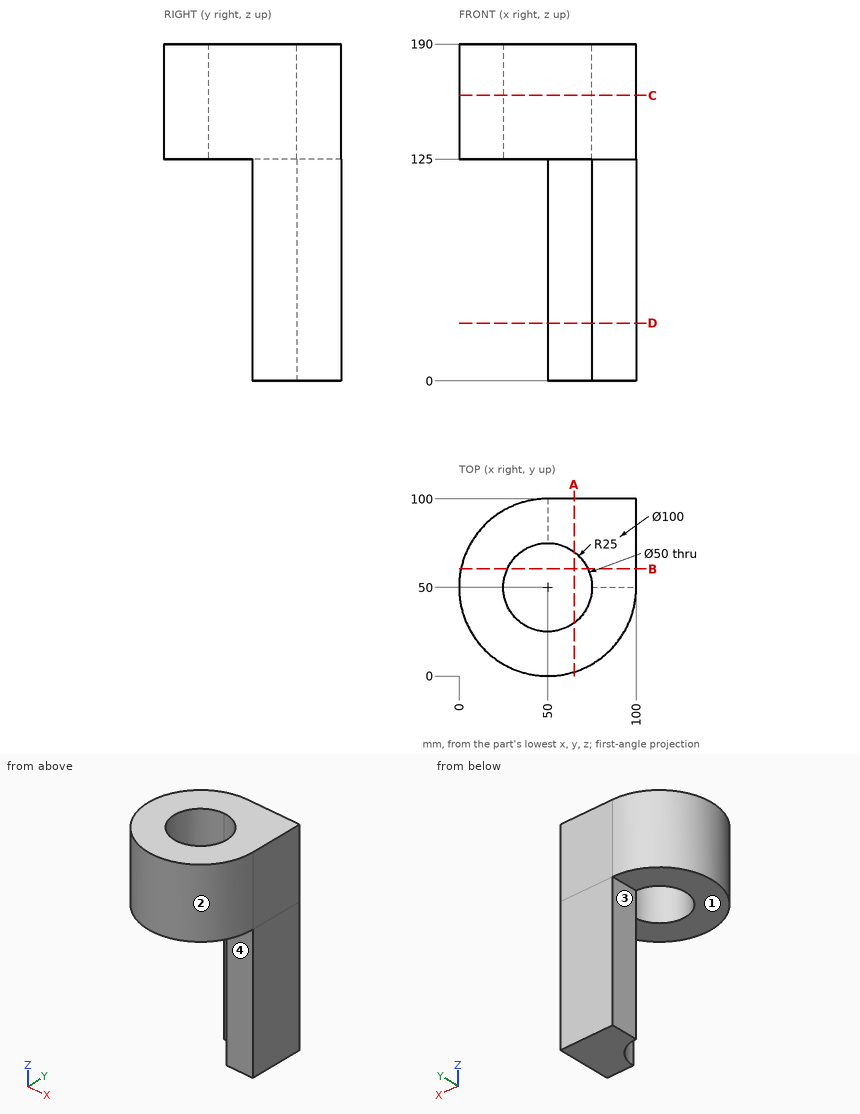
Could you check a few things on this drawing? It's one solid part, dimensions in mm from its lowest x, y, z. A direction names the side the tool comes from. Give positions to 0.01 mm unless a question says otherwise; leave off trailing zeros. Loops run counter-clockwise (first coordinate to the right, second up) from the corner with the lowest first, then second, coordinate; pieces in that order, holes last. Notation, with made-up numbers: M -29,-21 L -25,-21 A17 cw -25,-8 Z; hole C -36.75,85.5 d8. An arc over 180 degrees is marked long. Return JSON: item names as keys, results as strings.
Item 1: Imagine slicing it at D-D on z = 32.5. List the corners of the cut face in (x, y) for me.
A:
{"outline": "M 50,75 A25 cw 75,50 L 100,50 L 100,100 L 50,100 Z"}
Item 2: Imagine slicing it at B-B on y = 60.5. List the corners of the cut face in (x, z) for me, then the cut area to 3 significant figures.
A:
{"outline": "M 1.11,125 L 27.31,125 L 27.31,190 L 1.11,190 Z; M 72.69,0 L 100,0 L 100,190 L 72.69,190 Z", "area": "6,890 mm^2"}
Item 3: Imagine slicing it at C-C on z = 161. List the corners of the cut face in (x, y) for me, then the cut area to 3 significant figures.
A:
{"outline": "M 50,100 A50 ccw long 100,50 L 100,100 Z; hole C 50,50 d50", "area": "6,430 mm^2"}
Item 4: On a 3-axis mill with a long thin cutter (end or side, diameter ignored), from which of +Z, -Z, +X, -X, +Y, -Y can I reach the whole of each face in a straight line? I mean the marked faces 1, 2, 3 and 4. Say none if no direction works.
A:
{"face 1": "-Z, -X, -Y", "face 2": "+Z, -Z", "face 3": "-Z, -X, +Y, -Y", "face 4": "-Z, +X, -X, -Y"}
Item 5: I'm going to push flat-ended pins straight in: pin 1 Ø20 at (y, z) = (86, 56) entering from -X; pin 2 Ø12.5 at (x, z) = (91, 36.5) entering from -Y; pin 3 Ø1.5 at (x, y) = (45, 88) entering from -Z. Where does each tip first touch, or does it pass through?
A:
{"pin 1": "stops at x = 50", "pin 2": "stops at y = 50", "pin 3": "stops at z = 125"}
Item 6: Please list where these lines run through material, in increasing order: line 1 (X direction, y = 50, z = 175); line 2 (X direction, y = 79, z = 41).
A:
{"line 1": "x = 0 to 25, 75 to 100", "line 2": "x = 50 to 100"}
Item 7: Imagine slicing it at A-A on x = 65. List the corners of the cut face in (y, z) for me.
A:
{"outline": "M 2.3,125 L 30,125 L 30,190 L 2.3,190 Z; M 70,0 L 100,0 L 100,190 L 70,190 Z"}
